from build123d import *

# Parameters (mm, degrees)
F0_W     = 203.2
F0_H     = 200.025
F1_DEPTH = 3.175
F3_D     = 5.1054
F3_DEPTH = 25
F3_TIP   = 1.5338169022


# Not quite as in the source:
# - a length typed as a fraction of an inch, garbled in the dataset ("3 / 203.2 mm" for 3/8 in), is restored


with BuildPart() as f1:
    # F0 (on Front) → F1 (new body)
    with BuildSketch(Plane.XZ):
        Rectangle(F0_W, F0_H)
    extrude(amount=F1_DEPTH)

    # F3
    with Locations(Plane.XZ.offset(3.175)):
        with Locations((-72.7075, -49.2125), (72.7075, -49.2125), (-50.8, -71.12), (50.8, -71.12), (31.75, -47.625), (-11.1125, 66.675), (11.1125, 66.675)):
            Hole(F3_D / 2, depth=F3_DEPTH)
            with Locations((0, 0, -(F3_DEPTH + F3_TIP / 2))):  # 118° drill point
                Cone(0, F3_D / 2, F3_TIP, mode=Mode.SUBTRACT)


solid = f1.part
Verification items for the finished model (mm, model axes). Coordinates: 2 decimals unless noted, no trailing zeros. Order: outer loops, then holes, each group sorted by start corner. A loop starts at its lowest first (then second) coordinate and runs counter-clockwise, first axis right, second up.
1. Scan lines: line 1 (Z direction, x = -50.8, y = -0.6); line 2 (Z direction, x = 49.5, y = -2.35). Record each from-to range of solid material in increasing order.
Results found:
line 1: z = -100.01 to -73.67, -68.57 to 100.01
line 2: z = -100.01 to -73.32, -68.92 to 100.01
2. Sectioned sample at B-B, the plane x = -50.8. Record the cut outline in (y, z) (1 decimal).
Results found:
outline: (-3.2, -100) - (0, -100) - (0, -73.7) - (-3.2, -73.7) - close; (-3.2, -68.6) - (0, -68.6) - (0, 100) - (-3.2, 100) - close
3. Sectioned sample at A-A, the plane z = -71.12. Record the cut outline in (x, y) (3 decimals), and give its area (3 significant figures).
Results found:
outline: (-101.6, -3.175) - (-53.353, -3.175) - (-53.353, 0) - (-101.6, 0) - close; (-48.247, -3.175) - (48.247, -3.175) - (48.247, 0) - (-48.247, 0) - close; (53.353, -3.175) - (101.6, -3.175) - (101.6, 0) - (53.353, 0) - close
area: 613 mm2
4. Release check for a two-part mould opening along X. For faces 1 (the face through (-1, 0, 1)), 2 (the face through (49.622, -1.565, -73.385)) record: +X half, -X half, draft (parallel to the pull), parting line (faces both ways), or undercut.
Results found:
face 1: draft
face 2: undercut
5. Go/stop test with flat-tipped pins: pin 1 Ø6 at (x, z) = (50.8, -71.12) entering from +Y; pin 2 Ø2 at (x, z) = (-72.5, -49.5) entering from -Y. Record where each tip stops, or that it passes through.
Results found:
pin 1: stops at y = 0
pin 2: passes through
